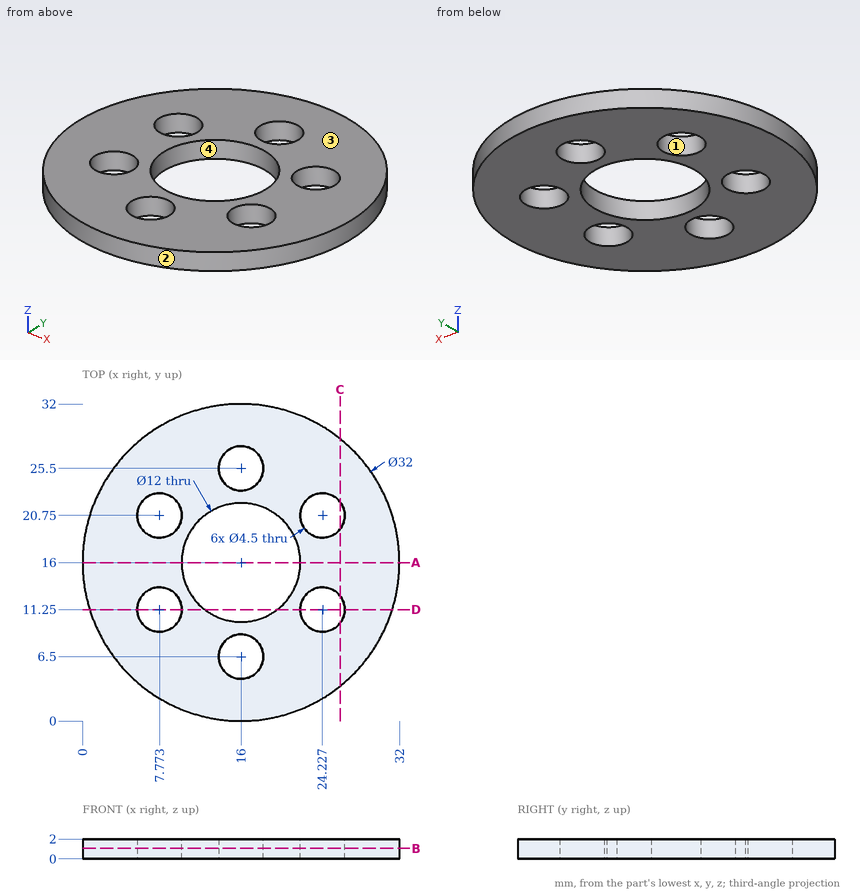
Here's the drawing with two shaded views (mm, measured from the low corner). I have some questions. Coordinates: 2 decimals unless noted, no trailing zeros. Write each loop counter-clockwise with the first axis right and the second up, starting at its lowest first coordinate (ties: lowest second). Pieces come first, ordered by that corner, then holes. Notation, with made-up numbers: M 57,69 L 66,69 A28 ccw 66,108 Z; hole C -37,-23.75 d10. An arc over 180 degrees is marked long. Write item = value, one per line. Start each with the question number.
Q1. If we section it at D-D, the plane y = 11.25: Write out the boundary of the cut face in (x, z).
Q2. Thinking about a two-plate mould opening in Y: for the marked faces 1, 2, 3 and 4, which applies, released by +Y, released by -Y, zero draft, split by the parting line, or undercut?
Q3. If we section it at A-A, the plane y = 16: Write out the boundary of the cut face in (x, z).
Q4. If I drill on L1, parallel to Y at x = 16, z = 1.05; L2, parallel to Y at x = 25, z = 1.5; L3, parallel to X at y = 11.5, z = 1 (1 decimal), over which ranges is the centre line in solid material (lowest first)? Write a range as [from, to].
Q5. If we section it at C-C, the plane x = 26: Write out the boundary of the cut face in (y, z).
Q6. If we section it at B-B, the plane z = 1.05: Write out the boundary of the cut face in (x, y), then the cut area to 3 significant figures.
Check sheet entries:
q1.outline = M 0.72,0 L 5.52,0 L 5.52,2 L 0.72,2 Z; M 10.02,0 L 12.33,0 L 12.33,2 L 10.02,2 Z; M 19.67,0 L 21.98,0 L 21.98,2 L 19.67,2 Z; M 26.48,0 L 31.28,0 L 31.28,2 L 26.48,2 Z
q2.face_1 = undercut
q2.face_2 = split by the parting line
q2.face_3 = zero draft
q2.face_4 = undercut
q3.outline = M 0,0 L 10,0 L 10,2 L 0,2 Z; M 22,0 L 32,0 L 32,2 L 22,2 Z
q4.L1 = [0, 4.25], [8.75, 10], [22, 23.25], [27.75, 32]
q4.L2 = [2.77, 9.14], [13.36, 18.64], [22.86, 29.23]
q4.L3 = [0.6, 5.5], [10, 12], [20, 22], [26.5, 31.4]
q5.outline = M 3.51,0 L 9.86,0 L 9.86,2 L 3.51,2 Z; M 12.64,0 L 19.36,0 L 19.36,2 L 12.64,2 Z; M 22.14,0 L 28.49,0 L 28.49,2 L 22.14,2 Z
q6.outline = C 16,16 d32; hole C 7.77,11.25 d4.5; hole C 7.77,20.75 d4.5; hole C 16,16 d12; hole C 16,6.5 d4.5; hole C 16,25.5 d4.5; hole C 24.23,11.25 d4.5; hole C 24.23,20.75 d4.5
q6.area = 596 mm²
